Geometry: final body of the model. Coordinates: model frame, mm. Coordinates: 2 decimals unless noted, no trailing zeros. Order: outer loops, then holes, each group sorted by start corner. A loop starts at its lowest first (then second) coordinate and runs counter-clockwise, first axis right, second up. Notation, with made-up numbers: (86.5, 59.5) - (91.5, 59.5) arc R31 cw to (91.5, 87.5) - close; hole circle Ø5 at (2.5, 73). An arc over 180 degrees is marked (long way). Use a Markdown table: item, result. Add a question column.
```python
from build123d import *

# Parameters (mm, degrees)
SKETCH1_R          = 3.25
SKETCH1_R_2        = 3.2639
BASE_FLANGE1_DEPTH = 3.175
CUT_EXTRUDE1_REACH = 56.837
SKETCH2_R          = 1.75


# Sheet-metal steps are written as plain solids
with BuildPart() as part:
    # Sketch1 → Base-Flange1 (new body)
    with BuildSketch(Plane(origin=(0, 0, 0), x_dir=(1, 0, 0), z_dir=(0, 1, 0))):
        with BuildLine():
            Line((9, 1.5), (9, 45))
            ThreePointArc((9, 45), (0, 54), (-9, 45))
            Line((-9, 45), (-9, 1.5))
            ThreePointArc((-9, 1.5), (0, -7.5), (9, 1.5))
        make_face()
        with Locations(Location((0, 0, 0), (0, 0, 270))):
            Circle(SKETCH1_R, mode=Mode.SUBTRACT)
        with Locations(Location((0, 45, 0), (0, 0, 270))):
            Circle(SKETCH1_R_2, mode=Mode.SUBTRACT)
    extrude(amount=-BASE_FLANGE1_DEPTH)

    # Sketch2 → Cut-Extrude1 (cut, up to next)
    with BuildSketch(Plane.XZ.offset(3.175), mode=Mode.PRIVATE) as cut_extrude1_sk1:
        with Locations(Location((0.05, -30.687503986, 0), (0, 0, 270))):
            Circle(SKETCH2_R)
    cut_extrude1_tool1 = extrude(cut_extrude1_sk1.sketch, amount=-CUT_EXTRUDE1_REACH, mode=Mode.PRIVATE) & part.part
    add(cut_extrude1_tool1.solids().sort_by_distance((0.05, -3.175, -30.687504))[0], mode=Mode.SUBTRACT)


solid = part.part
```
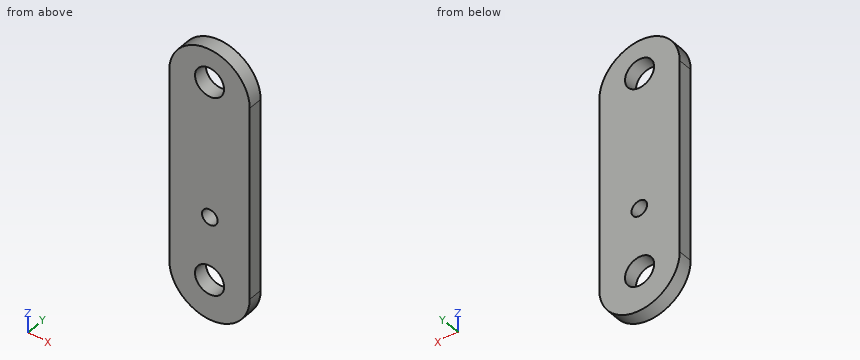
1) Section query B-B (z = -31). Return the cut outline in (x, y) (3 decimals).
2) Section query A-A (y = -2.65). Return the cut outline in (x, z).
3) Line query: line 1 (X direction, y = -1, z = -45); line 2 (Z direction, x = 2.5, y = -1.25); line 3 (X direction, y = -0.4, z = -1). Output: solid intervals per line, ascending. Write a range as from..to.
4) Section query D-D (z = 0). Return the cut outline in (x, y) (3 decimals), and give its area (3 significant figures).
5) First-contact query: pin 1 (1.5 mm diameter, centred on x = -3.5, y = -2.5, fed in from -Z). Flat tip, straight axial feed; report the tip coordinate or a pass-through.
6) Section query C-C (x = -2.5). Return the cut outline in (y, z) (3 decimals), and give its area (3 significant figures).
From the geometry:
| question | item | result |
|---|---|---|
| 1 | outline | (-9, -3.175) - (-1.672, -3.175) - (-1.672, 0) - (-9, 0) - close; (1.772, -3.175) - (9, -3.175) - (9, 0) - (1.772, 0) - close |
| 2 | outline | (-9, -45) arc R9 ccw to (9, -45) - (9, -1.5) arc R9 ccw to (-9, -1.5) - close; hole circle Ø6.53 at (0, -45); hole circle Ø6.5 at (0, 0); hole circle Ø3.5 at (0.05, -30.69) |
| 3 | line 1 | x = -9..-3.26, 3.26..9 |
| 3 | line 2 | z = -53.65..-47.1, -42.9..-2.08, 2.08..7.15 |
| 3 | line 3 | x = -8.99..-3.09, 3.09..8.99 |
| 4 | outline | (-8.874, -3.175) - (-3.25, -3.175) - (-3.25, 0) - (-8.874, 0) - close; (3.25, -3.175) - (8.874, -3.175) - (8.874, 0) - (3.25, 0) - close |
| 4 | area | 35.7 mm^2 |
| 5 | pin 1 | stops at z = -53.57 |
| 6 | outline | (-3.175, -53.646) - (0, -53.646) - (0, -47.098) - (-3.175, -47.098) - close; (-3.175, -42.902) - (0, -42.902) - (0, -2.077) - (-3.175, -2.077) - close; (-3.175, 2.077) - (0, 2.077) - (0, 7.146) - (-3.175, 7.146) - close |
| 6 | area | 167 mm^2 |
